CAD build for the part. Positions are in the model's coordinates, mm. A direction names the side the tool comes from. Coordinates: 2 decimals unless noted, no trailing zeros. Order: outer loops, then holes, each group sorted by start corner. A loop starts at its lowest first (then second) coordinate and runs counter-clockwise, first axis right, second up. Notation, with made-up numbers: (39.25, 43) -> (78.25, 43) arc R24 cw to (78.25, 76) -> close; hole circle Ø11 at (39.5, 14). An arc over 180 degrees is marked (long way). Use one line per item in the form item = value. Start each with the question number.
from build123d import *

# Parameters (mm, degrees)
SKETCH2_R          = 4.388085687
CUT_EXTRUDE1_DEPTH = 35
SKETCH4_R          = 12.137505268
CUT_EXTRUDE2_DEPTH = 19.362331983


with BuildPart() as part:
    # Sketch1 → Revolve1 (revolve)
    with BuildSketch(Plane.XY):
        Polygon((0, 0), (0, 153), (0.726418921, 153), (2.686091777, 128.637668017), (7.918657935, 128.637668017), (6.213660545, 107.320079818), (3.5, 103.794837091), (3.5, 55), (3.5, 53), (3.5, 0), align=None)
    revolve(axis=Axis((0, 0, 0), (0, 1, 0)))

    # Sketch2 → Cut-Extrude1 (cut)
    with BuildSketch(Plane.XZ):
        Circle(SKETCH2_R)
        Polygon((0, 3.5), (-3.031088913, 1.75), (-3.031088913, -1.75), (0, -3.5), (3.031088913, -1.75), (3.031088913, 1.75), align=None, mode=Mode.SUBTRACT)
    extrude(amount=-CUT_EXTRUDE1_DEPTH, mode=Mode.SUBTRACT)

    # Sketch4 → Cut-Extrude2 (cut, through all)
    with BuildSketch(Plane(origin=(0, 134.637668017, 0), x_dir=(1, 0, 0), z_dir=(0, 1, 0))):
        Circle(SKETCH4_R)
    extrude(amount=CUT_EXTRUDE2_DEPTH, mode=Mode.SUBTRACT)


solid = part.part
1) Cut at C-C on y = 119. Give the cut face in (x, z).
2) Cut at A-A on z = 0. Give the cut face in (x, y), then the cut area to 3 significant figures.
3) Cut at B-B on y = 44. Give the cut face in (x, z).
4) Probe L1, parallel to X at y = 17, z = -2.5; L2, parallel to X at y = 34.5, z = -1.5; L3, parallel to Y at x = 2.5, z = -1.25. List the from-to ranges inside material, lowest first.
5) 3-axis set-ups, long thin cutter, end or side, ignore diameter. For faces 1 (the face through (1.54, 17.26, 2.61)), 2 (the face through (3.233, 69.879, 1.341)), 3 (the face through (-1.49, 17.26, 2.64)): which of +Z, -Z, +X, -X, +Y, -Y reach the whole face in a straight line?
6) Drop flat-ended pins along their axis: P1, Ø1.5, axis at x = -5, z = -4.5, coming from the -Y side; P2, Ø2, axis at x = 3, y = 102.5, coming from the -Z side; P3, Ø8, axis at x = -2.5, y = 50, coming from the -Z side. Give the stop position or say it passes through.
Values follow:
q1.outline = circle Ø14.3 at (0, 0)
q2.outline = (-7.92, 128.64) -> (-6.21, 107.32) -> (-3.5, 103.79) -> (-3.5, 35) -> (-3.03, 35) -> (-3.03, 0) -> (3.03, 0) -> (3.03, 35) -> (3.5, 35) -> (3.5, 103.79) -> (6.21, 107.32) -> (7.92, 128.64) -> (2.69, 128.64) -> (2.2, 134.64) -> (-2.2, 134.64) -> (-2.69, 128.64) -> close
q2.area = 1,060 mm^2
q3.outline = circle Ø7 at (0, 0)
q4.L1 = -1.73 to 1.73
q4.L2 = -3.03 to 3.03
q4.L3 = 0 to 128.64
q5.face_1 = +Z, +X, -Y
q5.face_2 = -Y
q5.face_3 = +Z, -X, -Y
q6.P1 = 107.01
q6.P2 = -2.87
q6.P3 = -3.5
